Work out the finished part from the listing and answer in its coordinate system (mm). Round coordinates to 2 decimals unless told otherwise and drop trailing zeros. Order: outer loops, then holes, each group sorted by start corner. A loop starts at its lowest first (then second) coordinate and runs counter-clockwise, first axis right, second up. Notation, with made-up numbers: (68, 56) - (110, 56) arc R20 ccw to (110, 67) - close; hole circle Ø2 at (16, 59.25). An arc over 180 degrees is marked (long way). Use one line per item in the form item = value. Start each with the question number.
Q1. The part is cut by section C-C on x = 7.5. Determine the outline of the cut face in (y, z), plus the area to 3 significant figures.
Q2. The part is cut by section D-D on z = 36.5. Determine the outline of the cut face in (x, y), plus the area to 3 significant figures.
Q3. Find the intervals of material crossed by line 1 (Z direction, x = 8.5, y = -1); line 2 (Z direction, x = 11.25, y = -2.5); line 3 (X direction, y = -5, z = 10), in increasing order. Write a range as [from, to].
Q4. The part is cut by section B-B on z = 9. Determine the outline of the cut face in (x, y).
Q5. For a pull along Z with two mould halves and no side action, classify faces 1 (the cylindrical face through (16.33, -9.4, 40.32)), 2 (the flat face through (9, 0, 22)), 3 (the cylindrical face through (6.303, -9.141, 10.54)) as +Z half, -Z half, draft (parallel to the pull), parting line (faces both ways), or undercut.
Q6. The part is cut by section A-A on y = -14.5. Determine the outline of the cut face in (x, z) (3 decimals), plus the area to 3 significant figures.
from build123d import *

# Parameters (mm, degrees)
F0_W     = 19.05
F0_H     = 43.18
F1_DEPTH = 18.542
F2_R     = 9.525
F4_D     = 6.7564


with BuildPart() as f1:
    # F0 (on Front) → F1 (new body)
    with BuildSketch(Plane.XZ):
        with Locations((9.525, 21.59)):
            Rectangle(F0_W, F0_H)
    extrude(amount=F1_DEPTH)

    # F2
    f2_edges = [f1.edges().sort_by_distance(p)[0] for p in [
        (19.05, -9.271, 43.18),
    ]]
    fillet(f2_edges, radius=F2_R)

    # F4 (through all)
    with Locations(Plane.XZ.offset(18.542)):
        with Locations((9.525, 33.655), (9.525, 9.525)):
            Hole(F4_D / 2)


solid = f1.part
Found:
q1.outline = (-18.54, 0) - (0, 0) - (0, 6.82) - (-18.54, 6.82) - close; (-18.54, 12.23) - (0, 12.23) - (0, 30.95) - (-18.54, 30.95) - close; (-18.54, 36.36) - (0, 36.36) - (0, 43.18) - (-18.54, 43.18) - close
q1.area = 600 mm²
q2.outline = (0, -18.54) - (7.7, -18.54) - (7.7, 0) - (0, 0) - close; (11.35, -18.54) - (18.62, -18.54) - (18.62, 0) - (11.35, 0) - close
q2.area = 278 mm²
q3.line_1 = [0, 6.31], [12.74, 30.44], [36.87, 43.18]
q3.line_2 = [0, 6.62], [12.43, 30.75], [36.56, 43.02]
q3.line_3 = [0, 6.18], [12.87, 19.05]
q4.outline = (0, -18.54) - (6.19, -18.54) - (6.19, 0) - (0, 0) - close; (12.86, -18.54) - (19.05, -18.54) - (19.05, 0) - (12.86, 0) - close
q5.face_1 = +Z half
q5.face_2 = draft
q5.face_3 = undercut
q6.outline = (0, 0) - (19.05, 0) - (19.05, 33.655) arc R9.525 ccw to (9.525, 43.18) - (0, 43.18) - close; hole circle Ø6.756 at (9.525, 9.525); hole circle Ø6.756 at (9.525, 33.655)
q6.area = 731 mm²
